Could you check a few things on this drawing? It's one solid part, dimensions in mm from its lowest x, y, z. A direction names the side the tool comes from. Give positions to 0.01 mm unless a question says otherwise; leave off trailing zeros. Loops run counter-clockwise (first coordinate to the right, second up) from the corner with the lowest first, then second, coordinate; pieces in that order, holes last. Notation, with made-up numbers: M 79.25,34 L 111.25,34 A29 ccw 111.25,64 Z; hole C 18.5,29.5 d9. An arc over 180 degrees is marked long. Answer as CSV lines item,"result". Start each with the question number.
Item 1: I want a section at C-C on z = 10. List the corners of the cut face in (x, y) for me, plus the area to 3 significant figures.
Item 2: Will these pins go through, and if not, where does the flat tip stop? P1, Ø3, axis at x = 30.5, z = 5.5, coming from the +Y side; P2, Ø4, axis at x = 75.5, y = 44, coming from the -Z side; P3, Ø3, axis at x = 65, z = 5, coming from the +Y side; P4, Ø3, axis at y = 80, z = 10, coming from the +X side.
Item 3: I want a section at B-B on x = 45. List the corners of the cut face in (y, z) for me (1 decimal), plus the area to 3 significant figures.
Item 4: If we mould it in two halves opening along Y, with no side actions, what happens to the marked faces 1, 2 and 3? For each: released by +Y, released by -Y, zero draft, split by the parting line, or undercut.
Item 5: I want a section at D-D on x = 20. List the corners of the cut face in (y, z) for me, plus the area to 3 significant figures.
Item 6: For the marked faces 4, 5, 6, 7 and 8, which set-ups out of +Z, -Z, +X, -X, +Y, -Y let a thin tool reach every point of the face, with its end or its side?
Item 7: I want a section at A-A on y = 80. List the corners of the cut face in (x, z) for me, plus the area to 3 significant figures.
Item 8: If I drill on line 1 along Y through (x, z) = (43.25, 10); line 2 along X through (y, z) = (13.5, 6.75); line 3 along Y through (x, z) = (42, 10) (1 decimal), over which ranges is the centre line in solid material (lowest first)? Write a range as from..to.
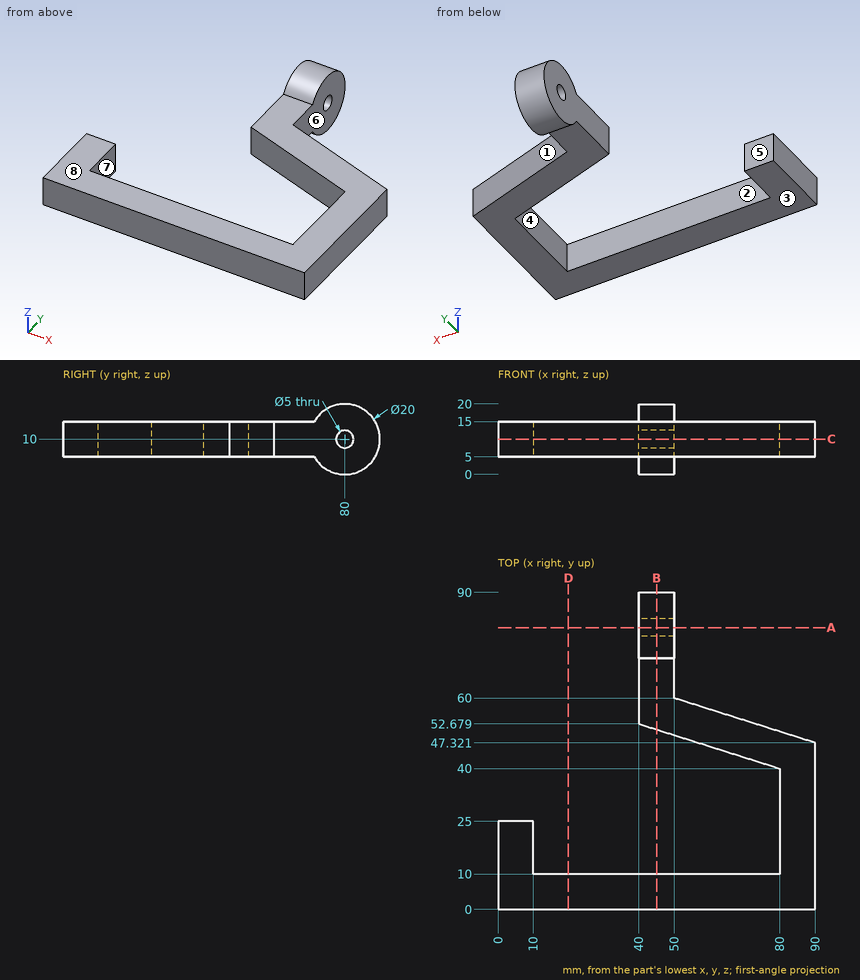
Result:
1,outline,"M 0,0 L 90,0 L 90,47.32 L 50,60 L 50,77.5 L 40,77.5 L 40,52.68 L 80,40 L 80,10 L 10,10 L 10,25 L 0,25 Z; M 40,82.5 L 50,82.5 L 50,90 L 40,90 Z"
1,area,"2,090 mm^2"
2,P1,"y = 10"
2,P2,"z = 5"
2,P3,"y = 55.72"
2,P4,"through"
3,outline,"M 0,5 L 10,5 L 10,15 L 0,15 Z; M 51.1,5 L 71.3,5 A10 ccw long 71.3,15 L 51.1,15 Z; hole C 80,10 d5"
3,area,"588 mm^2"
4,face 1,"released by +Y"
4,face 2,"undercut"
4,face 3,"zero draft"
5,outline,"M 0,5 L 10,5 L 10,15 L 0,15 Z"
5,area,"100 mm^2"
6,face 4,"+Z, -Z"
6,face 5,"+Z, -Z, -X, +Y"
6,face 6,"+Z, -Z, +X, +Y"
6,face 7,"+Z, -Z, +Y"
6,face 8,"+Z, +X, -X, -Y"
7,outline,"M 40,0 L 50,0 L 50,7.5 L 40,7.5 Z; M 40,12.5 L 50,12.5 L 50,20 L 40,20 Z"
7,area,"150 mm^2"
8,line 1,"0..10, 51.65..77.5, 82.5..90"
8,line 2,"0..10, 80..90"
8,line 3,"0..10, 52..77.5, 82.5..90"
